```python
from build123d import *

# Parameters (mm, degrees)
BOSS_EXTRUDE1_DEPTH              = 76.2
TAP_DRILL_FOR_M10X1_5_TAP1_D     = 8.5
TAP_DRILL_FOR_M10X1_5_TAP2_D     = 8.5
TAP_DRILL_FOR_M10X1_5_TAP2_DEPTH = 20
TAP_DRILL_FOR_M10X1_5_TAP2_TIP   = 2.553657631
FILLET1_R                        = 5


with BuildPart() as part:
    # Sketch1 → Boss-Extrude1 (new body)
    with BuildSketch(Plane(origin=(0, 0, 0), x_dir=(0, 0, -1), z_dir=(1, 0, 0))):
        Polygon((0, 0), (0, 50.8), (-6.35, 50.8), (-6.35, 6.35), (-50.8, 6.35), (-50.8, 0), align=None)
    extrude(amount=BOSS_EXTRUDE1_DEPTH)

    # Tap Drill for M10x1.5 Tap1 (through all)
    with Locations(Plane(origin=(0, 6.35, 0), x_dir=(1, 0, 0), z_dir=(0, 1, 0))):
        with Locations((25.4, -25.4), (50.8, -25.4)):
            Hole(TAP_DRILL_FOR_M10X1_5_TAP1_D / 2)

    # Tap Drill for M10x1.5 Tap2
    with Locations(Plane.XY.offset(6.35)):
        with Locations((25.4, 25.4), (50.8, 25.4)):
            Hole(TAP_DRILL_FOR_M10X1_5_TAP2_D / 2, depth=TAP_DRILL_FOR_M10X1_5_TAP2_DEPTH)
            with Locations((0, 0, -(TAP_DRILL_FOR_M10X1_5_TAP2_DEPTH + TAP_DRILL_FOR_M10X1_5_TAP2_TIP / 2))):  # 118° drill point
                Cone(0, TAP_DRILL_FOR_M10X1_5_TAP2_D / 2, TAP_DRILL_FOR_M10X1_5_TAP2_TIP, mode=Mode.SUBTRACT)

    # Fillet1
    fillet1_edges = [part.edges().sort_by_distance(p)[0] for p in [
        (38.1, 6.35, 6.35),
    ]]
    fillet(fillet1_edges, radius=FILLET1_R)


solid = part.part
```
Geometry check sheet. Reference: the model listing, model coordinates, mm. A direction names the side the tool comes from. Round coordinates to 2 decimals unless told otherwise and drop trailing zeros. Order: outer loops, then holes, each group sorted by start corner. A loop starts at its lowest first (then second) coordinate and runs counter-clockwise, first axis right, second up. Notation, with made-up numbers: M -14,-9 L 39,-9 A26 cw 39,5 Z; hole C 23.5,41.25 d4. An arc over 180 degrees is marked long. Answer as CSV lines item,"result".
1) Sectioned sample at D-D on z = 4. Record the cut outline in (x, y), and give its area (3 significant figures).
Entries:
outline,"M 0,0 L 76.2,0 L 76.2,50.8 L 0,50.8 Z; hole C 25.4,25.4 d8.5; hole C 50.8,25.4 d8.5"
area,"3,760 mm2"
2) Sectioned sample at A-A on x = 49. Record the cut outline in (y, z).
Entries:
outline,"M 0,0 L 21.55,0 L 21.55,6.35 L 11.35,6.35 A5 cw 6.35,11.35 L 6.35,21.55 L 0,21.55 Z; M 0,29.25 L 6.35,29.25 L 6.35,50.8 L 0,50.8 Z; M 29.25,0 L 50.8,0 L 50.8,6.35 L 29.25,6.35 Z"
3) Thickness scan on probe 1 along X at (y, z) = (2.25, 25.4); probe 2 along Z at (x, y) = (25.4, 4.75); probe 3 along Y at (x, z) = (35, 32). Record the ranges inside material, lowest first. Write a range as [from, to].
Entries:
probe 1,"[0, 21.15], [29.65, 46.55], [55.05, 76.2]"
probe 2,"[0, 21.15], [29.65, 50.8]"
probe 3,"[0, 6.35]"
4) Gauge pin test, flat ends, axial feed: pin 1 Ø5 at (y, z) = (13.5, 10) entering from +X; pin 2 Ø12 at (x, z) = (11.5, 41.5) entering from +Y; pin 3 Ø13.5 at (x, y) = (25.4, 25.4) entering from +Z. Record the tip position at first contact, or that the pin passes through.
Entries:
pin 1,"through"
pin 2,"y = 6.35"
pin 3,"z = 6.35"
5) Sectioned sample at C-C on z = 25.4. Record the cut outline in (x, y), and give its area (3 significant figures).
Entries:
outline,"M 0,0 L 21.15,0 L 21.15,6.35 L 0,6.35 Z; M 29.65,0 L 46.55,0 L 46.55,6.35 L 29.65,6.35 Z; M 55.05,0 L 76.2,0 L 76.2,6.35 L 55.05,6.35 Z"
area,"376 mm2"
6) Sectioned sample at B-B on y = 22. Record the cut outline in (x, z).
Entries:
outline,"M 0,0 L 22.85,0 L 22.85,6.35 L 0,6.35 Z; M 27.95,0 L 48.25,0 L 48.25,6.35 L 27.95,6.35 Z; M 53.35,0 L 76.2,0 L 76.2,6.35 L 53.35,6.35 Z"
7) Tool access check on faces 4 (the face through (38, 31, 6.35)), 5 (the face through (28.532, 28.272, 3.131)). Record the directions out of +Z, -Z, +X, -X, +Y, -Y that give a thin tool (end or side, any length) a straight path to the whole face; none if there is none.
Entries:
face 4,"+Z, +X, -X, +Y"
face 5,"+Z, -Z"
8) Mould release check, pull along Z, two halves, no side actions. Record for faces 1 (the face through (38, 6.35, 31)), 2 (the face through (46.746, 3.131, 24.123)), 3 (the face through (38, 3, 50.8)): +Z half, -Z half, draft (parallel to the pull), parting line (faces both ways), or undercut.
Entries:
face 1,"draft"
face 2,"undercut"
face 3,"+Z half"
